The figure shows three views and two pictorial views of one solid part (mm, origin at its lowest corner). Answer the questions. Coordinates: 2 decimals unless noted, no trailing zeros. Write each loop counter-clockwise with the first axis right and the second up, starting at its lowest first coordinate (ties: lowest second). Pieces come first, ordered by that corner, then holes. Notation, with made-up numbers: M -36.5,-3.75 L -17.5,-3.75 A8 ccw -17.5,2.25 Z; hole C 58,-40 d6. An arc over 180 degrees is marked long. Answer as CSV lines item,"result".
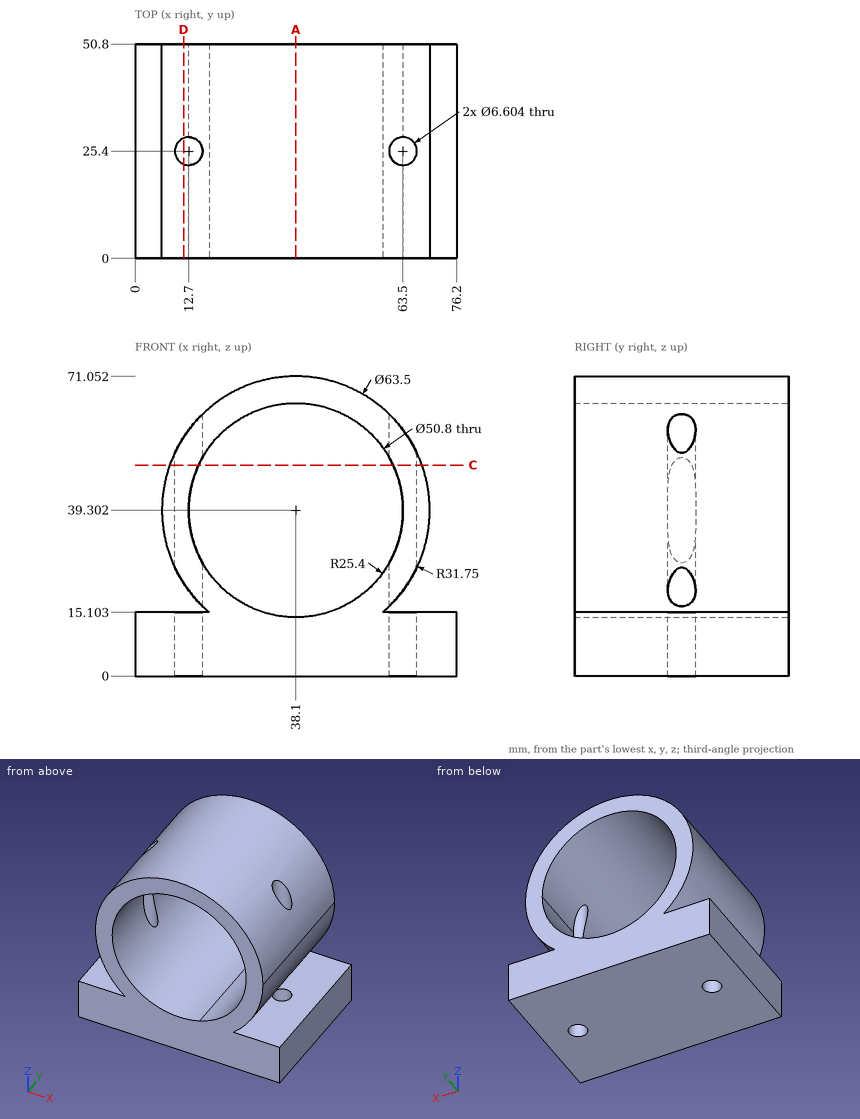
Q1. Find section C-C (z = 50). Give the vertices of the cut face in (x, y).
Output:
outline,"M 8.21,0 L 15.06,0 L 15.06,23.09 A3.3 cw long 15.06,27.71 L 15.06,50.8 L 8.21,50.8 Z; M 61.14,0 L 67.99,0 L 67.99,50.8 L 61.14,50.8 L 61.14,27.71 A3.3 cw long 61.14,23.09 Z"
Q2. Find section A-A (x = 38.1). Give the vertices of the cut face in (y, z).
Output:
outline,"M 0,0 L 50.8,0 L 50.8,13.9 L 0,13.9 Z; M 0,64.7 L 50.8,64.7 L 50.8,71.05 L 0,71.05 Z"
Q3. Find section D-D (x = 11.5). Give the vertices of the cut face in (y, z), and give its area (3 significant figures).
Output:
outline,"M 0,0 L 22.32,0 L 22.32,15.1 L 0,15.1 Z; M 0,21.97 L 22.32,21.97 L 22.32,56.64 L 0,56.64 Z; M 28.48,0 L 50.8,0 L 50.8,15.1 L 28.48,15.1 Z; M 28.48,21.97 L 50.8,21.97 L 50.8,56.64 L 28.48,56.64 Z"
area,"2,220 mm2"
Q4. Flat-ended cylindrical pins translate along their axes: pin 1 Ø1 at (y, z) = (26.5, 22) entering from -X; pin 2 Ø10.5 at (x, y) = (63.5, 25.4) entering from -Z; pin 3 Ø4 at (x, y) = (12.7, 25.4) entering from -Z; pin 4 Ø5 at (y, z) = (25.5, 27) entering from +X. Find the tip coordinate at first contact, or state that the pin passes through.
Output:
pin 1,"x = 15.59"
pin 2,"z = 0"
pin 3,"through"
pin 4,"x = 68.3"
Q5. Straight lines are drawn through the part: line 1 (Z direction, x = 37.5, y = 3.5) (1 decimal); line 2 (Y direction, x = 12.7, z = 46.5); line 3 (Z direction, x = 60, y = 46.5) (1 decimal). For each, find the intervals that lie inside material, in ascending order.
Output:
line 1,"0 to 13.9, 64.7 to 71"
line 2,"0 to 22.1, 28.7 to 50.8"
line 3,"0 to 15.1, 16.3 to 26.4, 52.2 to 62.3"
